from build123d import *
from OCP.BRepFilletAPI import BRepFilletAPI_MakeChamfer

# Parameters (mm, degrees)
SKETCH1_R           = 1.5
SKETCH1_R_2         = 4.75
BOSS_EXTRUDE1_DEPTH = 3
CHAMFER1_SIZE       = 0.2
CHAMFER2_SIZE       = 2
CHAMFER2_SIZE2      = 1.400415076


with BuildPart() as part:
    # Sketch1 → Boss-Extrude1 (new body)
    with BuildSketch(Plane(origin=(0, 0, 0), x_dir=(1, 0, 0), z_dir=(0, 1, 0))):
        with BuildLine():
            Line((-3.5, 7.5), (-3.5, 17))
            ThreePointArc((-3.5, 17), (0, 20.5), (3.5, 17))
            Line((3.5, 17), (3.5, 7.5))
            ThreePointArc((3.5, 7.5), (4.671572875, 4.671572875), (7.5, 3.5))
            Line((7.5, 3.5), (17, 3.5))
            ThreePointArc((17, 3.5), (20.5, 0), (17, -3.5))
            Line((17, -3.5), (7.5, -3.5))
            ThreePointArc((7.5, -3.5), (4.671572875, -4.671572875), (3.5, -7.5))
            Line((3.5, -7.5), (3.5, -17))
            ThreePointArc((3.5, -17), (0, -20.5), (-3.5, -17))
            Line((-3.5, -17), (-3.5, -7.5))
            ThreePointArc((-3.5, -7.5), (-4.671572875, -4.671572875), (-7.5, -3.5))
            Line((-7.5, -3.5), (-17, -3.5))
            ThreePointArc((-17, -3.5), (-20.5, 0), (-17, 3.5))
            Line((-17, 3.5), (-7.5, 3.5))
            ThreePointArc((-7.5, 3.5), (-4.671572875, 4.671572875), (-3.5, 7.5))
        make_face()
        with Locations(Location((0, 17, 0), (0, 0, 270))):
            Circle(SKETCH1_R, mode=Mode.SUBTRACT)
        with Locations(Location((0, 0, 0), (0, 0, 270))):
            Circle(SKETCH1_R_2, mode=Mode.SUBTRACT)
        with Locations(Location((17, 0, 0), (0, 0, 270))):
            Circle(SKETCH1_R, mode=Mode.SUBTRACT)
        with Locations(Location((0, -17, 0), (0, 0, 270))):
            Circle(SKETCH1_R, mode=Mode.SUBTRACT)
        with Locations(Location((-17, 0, 0), (0, 0, 270))):
            Circle(SKETCH1_R, mode=Mode.SUBTRACT)
        with Locations(Location((0, 9.5, 0), (0, 0, 270))):
            Circle(SKETCH1_R, mode=Mode.SUBTRACT)
        with Locations(Location((8, 0, 0), (0, 0, 270))):
            Circle(SKETCH1_R, mode=Mode.SUBTRACT)
        with Locations(Location((-8, 0, 0), (0, 0, 90))):
            Circle(SKETCH1_R, mode=Mode.SUBTRACT)
        with Locations(Location((0, -9.5, 0), (0, 0, 90))):
            Circle(SKETCH1_R, mode=Mode.SUBTRACT)
    extrude(amount=BOSS_EXTRUDE1_DEPTH)

    # Chamfer1
    chamfer1_edges = [part.edges().sort_by_distance(p)[0] for p in [
        (0, 0, -18.5),
        (0, 3, -18.5),
        (17, 0, -1.5),
        (17, 3, -1.5),
        (0, 0, 15.5),
        (0, 3, 15.5),
        (-17, 0, -1.5),
        (-17, 3, -1.5),
    ]]
    chamfer(chamfer1_edges, length=CHAMFER1_SIZE)

    # Chamfer2: one chamfer whose edges measure the first distance from different faces: ONE call of the kernel's chamfer builder (chamfer() names one face for all edges)
    chamfer2_edges_1 = [part.edges().sort_by_distance(p)[0] for p in [
        (0, 0, -11),
    ]]
    chamfer2_side_1 = [part.faces().sort_by_distance(p)[0] for p in [
        (0, 1.5, -11),
    ]]
    chamfer2_edges_2 = [part.edges().sort_by_distance(p)[0] for p in [
        (8, 0, -1.5),
    ]]
    chamfer2_side_2 = [part.faces().sort_by_distance(p)[0] for p in [
        (8, 1.5, -1.5),
    ]]
    chamfer2_edges_3 = [part.edges().sort_by_distance(p)[0] for p in [
        (-8, 0, 1.5),
    ]]
    chamfer2_side_3 = [part.faces().sort_by_distance(p)[0] for p in [
        (-8, 1.5, 1.5),
    ]]
    chamfer2_edges_4 = [part.edges().sort_by_distance(p)[0] for p in [
        (0, 0, 11),
    ]]
    chamfer2_side_4 = [part.faces().sort_by_distance(p)[0] for p in [
        (0, 1.5, 11),
    ]]
    chamfer2 = BRepFilletAPI_MakeChamfer(part.part.solid().wrapped)
    for e in chamfer2_edges_1:
        chamfer2.Add(CHAMFER2_SIZE, CHAMFER2_SIZE2, e.wrapped, chamfer2_side_1[0].wrapped)  # the first distance lies on this face
    for e in chamfer2_edges_2:
        chamfer2.Add(CHAMFER2_SIZE, CHAMFER2_SIZE2, e.wrapped, chamfer2_side_2[0].wrapped)  # the first distance lies on this face
    for e in chamfer2_edges_3:
        chamfer2.Add(CHAMFER2_SIZE, CHAMFER2_SIZE2, e.wrapped, chamfer2_side_3[0].wrapped)  # the first distance lies on this face
    for e in chamfer2_edges_4:
        chamfer2.Add(CHAMFER2_SIZE, CHAMFER2_SIZE2, e.wrapped, chamfer2_side_4[0].wrapped)  # the first distance lies on this face
    add(Compound.cast(chamfer2.Shape()), mode=Mode.REPLACE)


solid = part.part
Model file for the job. Use its own axes, mm. A direction names the side the tool comes from. Round coordinates to 2 decimals unless told otherwise and drop trailing zeros. Loops run counter-clockwise (first coordinate to the right, second up) from the corner with the lowest first, then second, coordinate; pieces in that order, holes last. Notation, with made-up numbers: (58, 44) -> (91, 44) arc R9 cw to (91, 59) -> close; hole circle Ø10 at (43, -31). An arc over 180 degrees is marked (long way). Answer as CSV lines item,"result". Start each with the question number.
1) Slice it at C-C (x = 13). List the corners of the cut face in (y, z), plus the area to 3 significant figures.
2) Slice it at A-A (z = 9.5). List the corners of the cut face in (x, y).
3) Pin check, flat tips, straight feed: P1, Ø1.8, axis at x = -8, z = 0, coming from the +Y side; P2, Ø0.9, axis at x = 10, y = 1, coming from the +Z side; P3, Ø1.5, axis at y = 1, z = 12.5, coming from the -X side; P4, Ø6, axis at x = 2, z = 1, coming from the -Y side. Stop position of each tip, or through.
4) Probe line 1 along X through (y, z) = (2.35, 17); line 2 along X through (y, z) = (1.5, 0); line 3 along X through (y, z) = (0.9, 0). List the from-to ranges inside material, lowest first.
5) Tool access for faces 5 (the face through (0.1, 1.5, 20.5)), 6 (the face through (-12, 1, -3.5)): list every direction of +Z, -Z, +X, -X, +Y, -Y with a clear straight run to the whole face (end or side of a thin tool).
6) Mould opens along Z. For faces 1 (the face through (-0.477, 1.875, 7.986)), 2 (the face through (4.703, 1.479, 4.641)), 3 (the face through (-1, 3, -5)), 4 (the face through (20.5, 1.5, -0.1)) say: +Z half, -Z half, draft (parallel to the pull), parting line (faces both ways), or undercut.
7) Slice it at B-B (y = 0.8). State how many separate pieces and enclosed holes the cut face has, plus the area to 3 significant figures.
Filled in:
1,outline,"(0, -3.5) -> (3, -3.5) -> (3, 3.5) -> (0, 3.5) -> close"
1,area,"21.0 mm2"
2,outline,"(-3.5, 0) -> (-2.9, 0) -> (-1.5, 2) -> (-1.5, 3) -> (-3.5, 3) -> close; (1.5, 2) -> (2.9, 0) -> (3.5, 0) -> (3.5, 3) -> (1.5, 3) -> close"
3,P1,"passes through"
3,P2,"stops at z = 3.5"
3,P3,"stops at x = -3.5"
3,P4,"stops at y = 0"
4,line 1,"x = -3.5 to -1.5, 1.5 to 3.5"
4,line 2,"x = -20.5 to -18.5, -15.5 to -9.85, -6.15 to -4.75, 4.75 to 6.15, 9.85 to 15.5, 18.5 to 20.5"
4,line 3,"x = -20.5 to -18.5, -15.5 to -10.27, -5.73 to -4.75, 4.75 to 5.73, 10.27 to 15.5, 18.5 to 20.5"
5,face 5,"+Z, +Y, -Y"
5,face 6,"-Z, -X, +Y, -Y"
6,face 1,"undercut"
6,face 2,"+Z half"
6,face 3,"draft"
6,face 4,"parting line"
7,separate pieces,"1"
7,enclosed holes,"9"
7,area,"350 mm2"
